Drawing for the job (mm, zero at the part's lowest x, y, z). A direction names the side the tool comes from. Round coordinates to 2 decimals unless told otherwise and drop trailing zeros. Write each loop counter-clockwise with the first axis right and the second up, starting at its lowest first coordinate (ties: lowest second). Pieces come first, ordered by that corner, then holes. Notation, with made-up numbers: (88, 78) - (112, 78) arc R18 cw to (112, 84) - close; hole circle Ø8 at (-29.5, 36.25). An arc over 180 degrees is marked (long way). Answer in a Markdown table with one row per item.
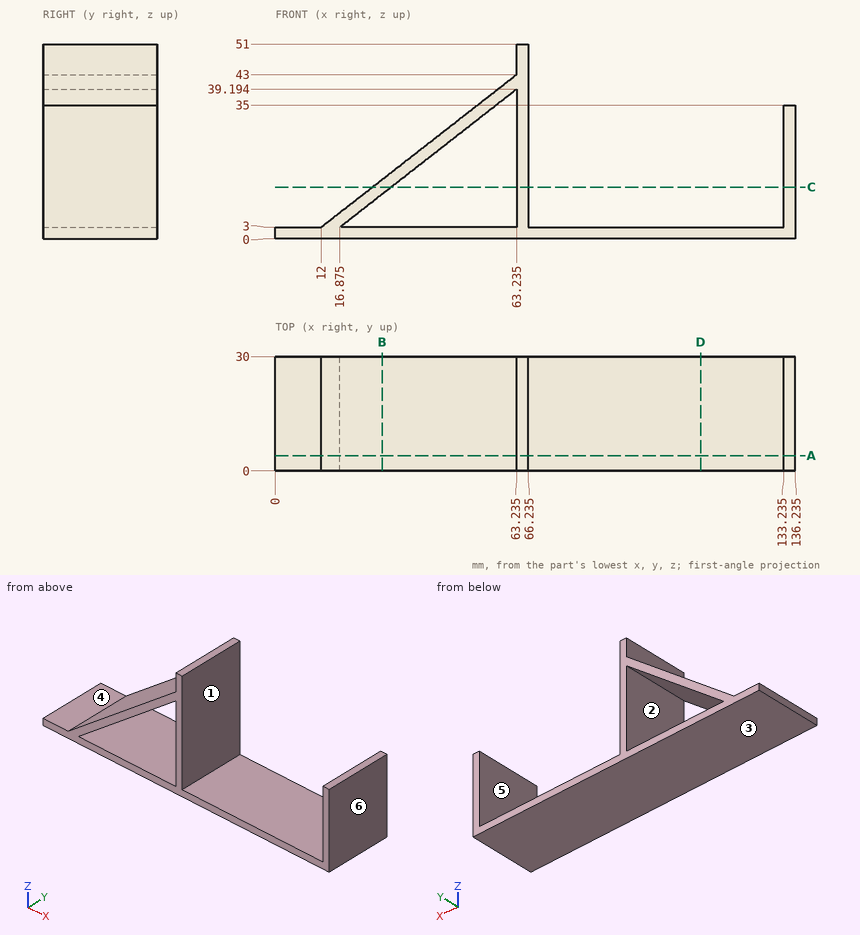
Q1. Saw through at C-C on z = 13.5. List the corners of the cut face in (x, y) (1 decimal), then the cut area to 3 significant figures.
Computed:
| item | result |
|---|---|
| outline | (25.4, 0) - (30.3, 0) - (30.3, 30) - (25.4, 30) - close; (63.2, 0) - (66.2, 0) - (66.2, 30) - (63.2, 30) - close; (133.2, 0) - (136.2, 0) - (136.2, 30) - (133.2, 30) - close |
| area | 326 mm2 |
Q2. Flat gauge pins, fed straight in: pin 1 (8 mm diameter, centred on y = 7, z = 41, fed in from -X); pin 2 (2 mm diameter, centred on x = 44.5, y = 8.5, fed in from +Z); pin 3 (6 mm diameter, centred on x = 8.5, y = 19, fed in from +Z); pin 4 (1 mm diameter, centred on x = 107.5, y = 26, fed in from -Z). Where does each tip first touch, or does it go through?
Computed:
| item | result |
|---|---|
| pin 1 | stops at x = 55.55 |
| pin 2 | stops at z = 29.15 |
| pin 3 | stops at z = 3 |
| pin 4 | stops at z = 0 |
Q3. Saw through at B-B on x = 28. List the corners of the cut face in (y, z), then the cut area to 3 significant figures.
Computed:
| item | result |
|---|---|
| outline | (0, 0) - (30, 0) - (30, 3) - (0, 3) - close; (0, 11.69) - (30, 11.69) - (30, 15.49) - (0, 15.49) - close |
| area | 204 mm2 |
Q4. Saw through at A-A on y = 4. List the corners of the cut face in (x, z) (1 decimal).
Computed:
| item | result |
|---|---|
| outline | (0, 0) - (136.2, 0) - (136.2, 35) - (133.2, 35) - (133.2, 3) - (66.2, 3) - (66.2, 51) - (63.2, 51) - (63.2, 43) - (12, 3) - (0, 3) - close; hole (16.9, 3) - (63.2, 3) - (63.2, 39.2) - close |
Q5. Saw through at D-D on x = 111.5. List the corners of the cut face in (y, z).
Computed:
| item | result |
|---|---|
| outline | (0, 0) - (30, 0) - (30, 3) - (0, 3) - close |
Q6. Pull direction X, two halves, no side cores. Call the marked faces 4, 5 and 6: released by +X, released by -X, zero draft, split by the parting line, or undercut.
Computed:
| item | result |
|---|---|
| face 4 | zero draft |
| face 5 | undercut |
| face 6 | released by +X |
Q7. 3-axis set-ups, long thin cutter, end or side, ignore diameter. For the marked faces 1, 2 and 3: which of +Z, -Z, +X, -X, +Y, -Y reach the whole face in a straight line?
Computed:
| item | result |
|---|---|
| face 1 | +Z, +Y, -Y |
| face 2 | +Y, -Y |
| face 3 | -Z, +X, -X, +Y, -Y |
Q8. Drill centre lines: line 1 (X direction, y = 18, z = 31.5) (1 decimal); line 2 (X direction, y = 23.5, z = 33.5) (1 decimal); line 3 (Z direction, x = 80, y = 4.5). Where is each one in solid material? Low to high.
Computed:
| item | result |
|---|---|
| line 1 | x = 48.5 to 53.4, 63.2 to 66.2, 133.2 to 136.2 |
| line 2 | x = 51.1 to 55.9, 63.2 to 66.2, 133.2 to 136.2 |
| line 3 | z = 0 to 3 |
